Autodesk Inventor part; units mm, degrees
ref_plane "YZ Plane" through (0, 0, 0) normal (1, 0, 0) x (0, 1, 0)
ref_plane "XZ Plane" through (0, 0, 0) normal (0, 1, 0) x (-1, 0, 0)
ref_plane "XY Plane" through (0, 0, 0) normal (0, 0, 1) x (1, 0, 0)
sketch "Sketch1" plane through (0, 0, 0) normal (0, 0, 1) x (1, 0, 0)
  circle A0 centre (8.7249, -8.7376) radius 1.2573
  circle A1 centre (8.7249, -8.7376) radius 2.3876
  dimension "d0" = 4.7752
extrude "Extrusion1" add sketch "Sketch1" along normal mid plane 11.176 contours A0 | A1
sketch "Sketch2" plane through (8.7249, -8.7376, 5.588) normal (0, 0, 1) x (1, 0, 0)
  circle A0 centre (0, 0) radius 1.2573
extrude "Extrusion2" add sketch "Sketch2" along normal blind 2.1844
mirror "Mirror1" about plane through (0, 0, 0) normal (0, 0, 1) of "Extrusion2"
chamfer "Chamfer1" distance 0.127 angle 45 4 edges at (7.4676, -8.7376, 7.7724) (6.3373, -8.7376, 5.588) (6.3373, -8.7376, -5.588) (7.4676, -8.7376, -7.7724)
properties part number "Channel - Hinge Pin" material "Steel, Mild"
For this review, take the finished solid that the model builds, in its own axes (mm). A direction names the side the tool comes from. Give positions to 0.01 mm unless a question says otherwise; leave off trailing zeros. Order: outer loops, then holes, each group sorted by start corner. A loop starts at its lowest first (then second) coordinate and runs counter-clockwise, first axis right, second up. Notation, with made-up numbers: (-26.75, 29.25) - (10.25, 29.25) arc R30 cw to (10.25, 64.25) - close; hole circle Ø5 at (22.25, -20). An arc over 180 degrees is marked (long way). Answer as a JSON object with one key per item and string values. Group by question number.
Item 1: Take a section at A-A on z = -4.75. Give the boundary of the cut face in (x, y).
Item 2: Wall thickness on line 1 along Z through (x, y) = (10.75, -7.9); line 2 along X through (y, z) = (-8.1, -5.5); line 3 along Y through (x, z) = (9.45, -2): over which ranges is each line inside the solid? List them lowest first.
Item 3: Clearance check with flat-ended pins moving along their axes: pin 1 Ø1 at (y, z) = (-10, -0.5) entering from +X; pin 2 Ø2 at (y, z) = (-7.5, 6) entering from -X. State where each tip first meets the part, or that it passes through.
Item 4: Take a section at B-B on z = 6. Give the boundary of the cut face in (x, y).
Item 5: Machinability: for faces 1 (the cylindrical face through (6.34, -8.63, 0.08)), 2 (the flat face through (10, -10, 5.588)), 3 (the cylindrical face through (9.924, -8.36, -6.602)), which of the approach directions +Z, -Z, +X, -X, +Y, -Y give a long, thin tool a straight path to every point of the face, cutting with its end or side? Answer none if there is none.
Reported:
{
 "1": {"outline": "circle Ø4.78 at (8.72, -8.74)"},
 "2": {"line 1": "-5.59 to 5.59", "line 2": "6.46 to 10.99", "line 3": "-11.01 to -6.46"},
 "3": {"pin 1": "x = 10.99", "pin 2": "x = 6.37"},
 "4": {"outline": "circle Ø2.51 at (8.72, -8.74)"},
 "5": {"face 1": "+Z, -Z", "face 2": "+Z", "face 3": "-Z"}
}
